Input: dimensioned drawing with shaded views. Units: mm. Origin: part minimum x, y, z. A direction names the side the tool comes from. Round coordinates to 2 decimals unless told otherwise and drop trailing zeros. Write each loop counter-clockwise with the first axis right and the second up, starting at its lowest first coordinate (ties: lowest second). Pieces come first, ordered by that corner, then holes. Notation, with made-up numbers: (74, 38.25) - (86, 38.25) arc R19 cw to (86, 46.25) - close; hole circle Ø8 at (10.5, 83). An arc over 180 degrees is marked (long way). Use one line per item in the form item = value.
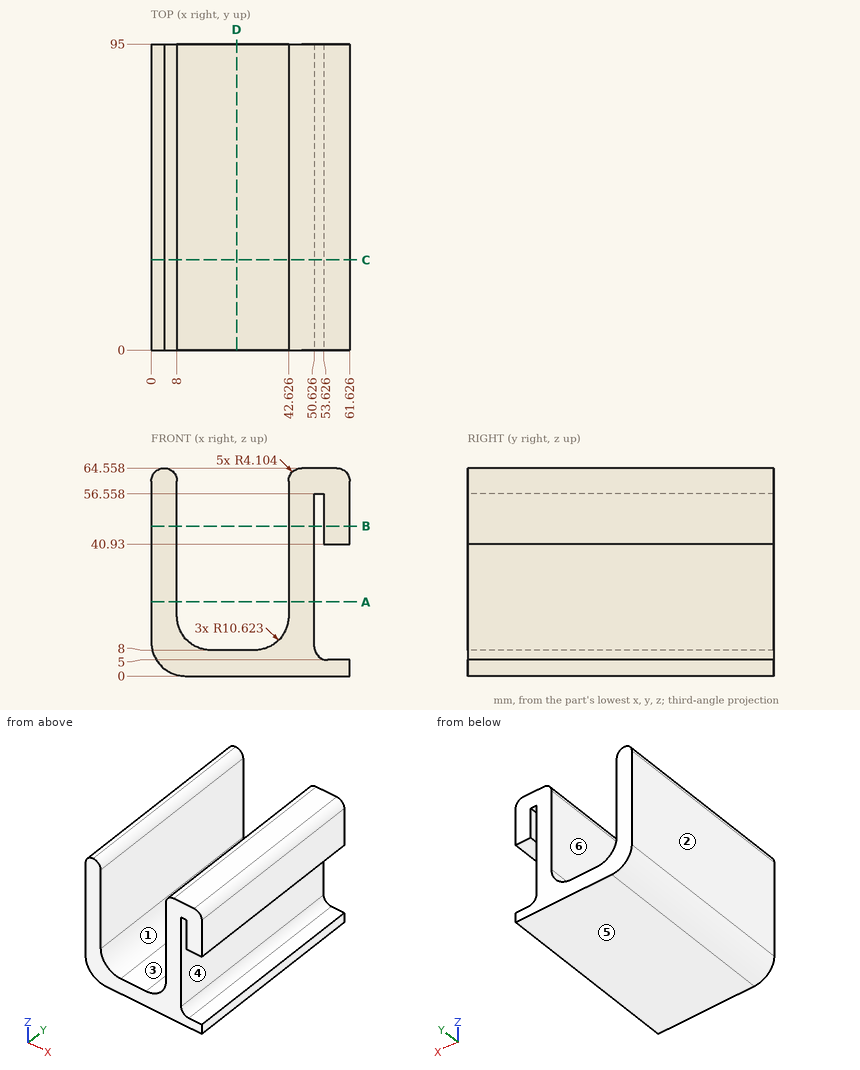
(1) Cut plane B-B on z = 46.5. Output: boundary loops of the cut face in (x, y).
Derived:
outline = (0, 0) - (8, 0) - (8, 95) - (0, 95) - close; (42.63, 0) - (50.63, 0) - (50.63, 95) - (42.63, 95) - close; (53.63, 0) - (61.63, 0) - (61.63, 95) - (53.63, 95) - close
(2) Cut plane C-C on y = 28. Output: boundary loops of the cut face in (x, z) (1 decimal), then the cut area to 3 significant figures.
Derived:
outline = (0, 10.6) arc R10.6 ccw to (10.6, 0) - (61.6, 0) - (61.6, 5) - (54.7, 5) arc R4.1 cw to (50.6, 9.1) - (50.6, 56.6) - (53.6, 56.6) - (53.6, 40.9) - (61.6, 40.9) - (61.6, 60.5) arc R4.1 ccw to (57.5, 64.6) - (46.7, 64.6) arc R4.1 ccw to (42.6, 60.5) - (42.6, 18.6) arc R10.6 cw to (32, 8) - (18.6, 8) arc R10.6 cw to (8, 18.6) - (8, 60.5) arc R4.1 ccw to (4, 64.6) arc R4.1 ccw to (0, 60.5) - close
area = 1,590 mm^2
(3) First-contact query: pin 1 Ø8 at (x, y) = (26, 70.5) entering from +Z. Flat tip, straight axial feed; report the tip coordinate or a pass-through.
Derived:
pin_1 = 8
(4) Material intervals for L1, parallel to X at y = 89, z = 51; L2, parallel to X at y = 58.5, z = 32.5; L3, parallel to X at y = 13.5, z = 57.5, sorted ascending.
Derived:
L1 = 0 to 8, 42.63 to 50.63, 53.63 to 61.63
L2 = 0 to 8, 42.63 to 50.63
L3 = 0 to 8, 42.63 to 61.63
(5) Cut plane A-A on z = 23. Output: boundary loops of the cut face in (x, y), then the cut area to 3 significant figures.
Derived:
outline = (0, 0) - (8, 0) - (8, 95) - (0, 95) - close; (42.63, 0) - (50.63, 0) - (50.63, 95) - (42.63, 95) - close
area = 1,520 mm^2
(6) Draft query along Z for the marked faces 3, 4, 5 and 6. Return one class per face: released by +Z, released by -Z, zero draft, split by the parting line, or undercut.
Derived:
face_3 = released by +Z
face_4 = undercut
face_5 = released by -Z
face_6 = zero draft
(7) Cut plane D-D on x = 26.5. Output: boundary loops of the cut face in (y, z), then the cut area to 3 significant figures.
Derived:
outline = (0, 0) - (95, 0) - (95, 8) - (0, 8) - close
area = 760 mm^2
(8) Access query for the marked faces 1 and 2. Directions: +Z, -Z, +X, -X, +Y, -Y. A direction counts if a zero-diameter tool reaches every point of the face in a straight line with its end or side. Return the directions, or none.
Derived:
face_1 = +Z, +Y, -Y
face_2 = +Z, -Z, -X, +Y, -Y
